from build123d import *

# Parameters (mm, degrees)
F0_W     = 25.3138970584
F0_H     = 25.3138970584
F0_W_2   = 25.5399178714
F0_H_2   = 25.9919501841
F0_W_3   = 25.5399160087
F1_DEPTH = 25.4
F2_W     = 25.5080536008
F2_H     = 25.2275522798
F3_DEPTH = 25.4


with BuildPart() as f1:
    # F0 (on Top) → F1 (new body)
    with BuildSketch(Plane.XY):
        with Locations((12.6569485292, 12.6569485292)):
            Rectangle(F0_W, F0_H)
        with Locations((38.083855994, 12.6569485292)):
            Rectangle(F0_W_2, F0_H)
        with Locations((38.083855994, -12.9959750921)):
            Rectangle(F0_W_2, F0_H_2)
        with Locations((-12.7699580044, -12.9959750921)):
            Rectangle(F0_W_3, F0_H_2)
        with Locations((-12.7699580044, 12.6569485292)):
            Rectangle(F0_W_3, F0_H)
    extrude(amount=F1_DEPTH)

    # F2 (on Front) → F3 (join)
    with BuildSketch(Plane.XZ):
        with Locations((-12.7540268004, 37.929170765)):
            Rectangle(F2_W, F2_H)
    extrude(amount=F3_DEPTH)


solid = f1.part
Check sheet for the modelled part. Datum: model origin and axes. Units: mm. A direction names the side the tool comes from. Give positions to 0.01 mm unless a question says otherwise; leave off trailing zeros. Loops run counter-clockwise (first coordinate to the right, second up) from the corner with the lowest first, then second, coordinate; pieces in that order, holes last. Notation, with made-up numbers: M -17,48 L 13,48 A18 cw 13,52 Z; hole C -20,20 d5. An arc over 180 degrees is marked long. Use a Markdown table: item, result. Add a question column.
Q1. Go/stop test with flat-tipped pins: pin 1 (5 mm diameter, centred on y = 0.5, z = 39.5, fed in from +X); pin 2 (20.5 mm diameter, centred on x = 19, z = 8, fed in from -Y); pin 3 (7.5 mm diameter, centred on x = -13, z = 43.5, fed in from -Y); pin 4 (7.5 mm diameter, centred on y = -13.5, z = 43, fed in from -X). Record where each tip stops, or that it passes through.
Q2. Sectioned sample at C-C, the plane x = -13. Record the cut outline in (y, z).
Q3. Scan lines: line 1 along X through (y, z) = (-19, 17); line 2 along Z through (x, y) = (17, 19.5); line 3 along Y through (x, z) = (-19, 48). Record each from-to range of solid material in increasing order. Write a range as [from, to].
Q4. Sectioned sample at B-B, the plane z = 5. Record the cut outline in (x, y), then the cut area to 3 significant figures.
Q5. Tool access check on faces 4 (the flat face through (-13, -25.4, 38)), 5 (the flat face through (0, -13, 25)), 6 (the flat face through (-13, 0, 38)). Record the directions out of +Z, -Z, +X, -X, +Y, -Y that give a thin tool (end or side, any length) a straight path to the whole face; none if there is none.
Q6. Sectioned sample at D-D, the plane y = 11. Record the cut outline in (x, z), then the cut area to 3 significant figures.
Q7. Mould release check, pull along X, two halves, no side actions. Record for faces 1 (the flat face through (-25.54, 0, 13)), 2 (the flat face through (50.854, -1, 13)), 3 (the flat face through (25.314, -13, 13)): pulls with the +X half, pulls with the -X half, needs draft (parallel to the pull), parting line crosses it, or undercut.
Verdict:
| question | item | result |
|---|---|---|
| 1 | pin 1 | x = 0 |
| 1 | pin 2 | y = -25.99 |
| 1 | pin 3 | y = -25.4 |
| 1 | pin 4 | x = -25.51 |
| 2 | outline | M -25.99,0 L 25.31,0 L 25.31,25.4 L 0,25.4 L 0,50.54 L -25.4,50.54 L -25.4,25.4 L -25.99,25.4 Z |
| 3 | line 1 | [-25.54, 0], [25.31, 50.85] |
| 3 | line 2 | [0, 25.4] |
| 3 | line 3 | [-25.4, 0] |
| 4 | outline | M -25.54,-25.99 L 0,-25.99 L 0,0 L 25.31,0 L 25.31,-25.99 L 50.85,-25.99 L 50.85,25.31 L -25.54,25.31 Z |
| 4 | area | 3,260 mm^2 |
| 5 | face 4 | +Z, +X, -X, -Y |
| 5 | face 5 | +Z, -Z, -Y |
| 5 | face 6 | +Z, +X, -X, +Y |
| 6 | outline | M -25.54,0 L 50.85,0 L 50.85,25.4 L -25.54,25.4 Z |
| 6 | area | 1,940 mm^2 |
| 7 | face 1 | pulls with the -X half |
| 7 | face 2 | pulls with the +X half |
| 7 | face 3 | undercut |
